CAD build for the part. Positions are in the model's coordinates, mm. Face numbers are marked on the shaded views. A direction names the side the tool comes from. Give positions to 0.01 mm unless a question says otherwise; leave off trailing zeros. Order: outer loops, then holes, each group sorted by start corner. A loop starts at its lowest first (then second) coordinate and runs counter-clockwise, first axis right, second up. Notation, with made-up numbers: (53, -26.5) -> (99, -26.5) arc R34 cw to (99, 6.5) -> close; hole circle Ø2 at (-37, -36). An arc over 180 degrees is marked (long way). Use one line per item in the form item = value. Start each with the question number.
1) Mould opens along Z. For the marked faces 4 and 5 say: pulls with the +Z half, pulls with the -Z half, needs draft (parallel to the pull), parting line crosses it, or undercut.
2) Cut at C-C, the plane x = 14.5. Give the cut face in (y, z).
3) Cut at D-D, the plane y = -45. Give the cut face in (x, z), and give its area (3 significant figures).
4) Probe line 1 (X direction, y = -50, z = 0); line 2 (Y direction, x = 14, z = 0); line 3 (X direction, y = 47.5, z = 1.5). List the from-to ranges inside material, lowest first.
5) Tool access for the marked faces 1, 2 and 3: list every direction of +Z, -Z, +X, -X, +Y, -Y with a clear straight run to the whole face (end or side of a thin tool).
6) Cut at B-B, the plane y = 16.5. Give the cut face in (x, z), and give its area (3 significant figures).
7) Drop flat-ended pins along their axis: P1, Ø8, axis at x = 81, y = -26, coming from the +Z side; P2, Ø6, axis at x = 52, y = 50.5, coming from the -Z side; P3, Ø6, axis at y = -35.5, z = -18.5, coming from the -X side. Give the stop position or say it passes through.
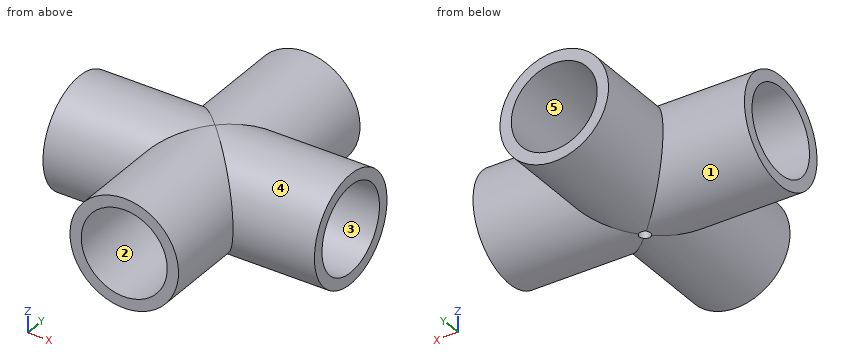
from build123d import *

# Parameters (mm, degrees)
SKETCH1_R                = 30.48
SKETCH1_R_2              = 24.13
BOSS_EXTRUDE1_DEPTH      = 152.4
BOSS_EXTRUDE2_DEPTH      = 76.2
BOSS_EXTRUDE2_DEPTH_BACK = 76.2
SKETCH2_R                = 30.48
SKETCH2_R_2              = 24.13
SKETCH4_R                = 3.175
CUT_EXTRUDE1_DEPTH       = 174.093126512


with BuildPart() as part:
    # Sketch1 → Boss-Extrude1 (new body)
    with BuildSketch(Plane(origin=(0, 0, 0), x_dir=(0, 0, -1), z_dir=(1, 0, 0))):
        with Locations(Location((0, 0, 0), (0, 0, 180))):
            Circle(SKETCH1_R)
        with Locations(Location((0, 0, 0), (0, 0, 180))):
            Circle(SKETCH1_R_2, mode=Mode.SUBTRACT)
    extrude(amount=BOSS_EXTRUDE1_DEPTH)

    # Sketch2 → Boss-Extrude2 (add, two sides: drawn at the far end of the back side and taken through both)
    with BuildSketch(Plane(origin=(0, 0, 0), x_dir=(1, 0, 0), z_dir=(0, 1, 0)).offset(-BOSS_EXTRUDE2_DEPTH_BACK)):
        with Locations(Location((76.2, 0, 0), (0, 0, 270))):
            Circle(SKETCH2_R)
        with Locations(Location((76.2, 0, 0), (0, 0, 270))):
            Circle(SKETCH2_R_2, mode=Mode.SUBTRACT)
    extrude(amount=BOSS_EXTRUDE2_DEPTH + BOSS_EXTRUDE2_DEPTH_BACK)

    # Sketch4 → Cut-Extrude1 (cut, through all)
    with BuildSketch(Plane.XY):
        with Locations(Location((76.2, 0, 0), (0, 0, 44.999999719))):
            Circle(SKETCH4_R)
    extrude(amount=-CUT_EXTRUDE1_DEPTH, mode=Mode.SUBTRACT)


solid = part.part
Result:
q1.face_4 = parting line crosses it
q1.face_5 = undercut
q2.outline = circle Ø60.96 at (0, 0); hole circle Ø48.26 at (0, 0)
q3.outline = circle Ø60.96 at (76.2, 0); hole circle Ø48.26 at (76.2, 0)
q3.area = 1,090 mm²
q4.line_1 = 45.72 to 52.07, 100.33 to 106.68
q4.line_2 = -30.48 to -24.13, 24.13 to 30.48
q4.line_3 = 45.76 to 52.12, 100.28 to 106.64
q5.face_1 = -X
q5.face_2 = -Y
q5.face_3 = +X
q6.outline = (0, -25.63) -> (59.7, -25.63) arc R30.48 ccw to (92.7, -25.63) -> (152.4, -25.63) -> (152.4, -17.61) -> (101.08, -17.61) arc R30.48 ccw to (101.08, 17.61) -> (152.4, 17.61) -> (152.4, 25.63) -> (92.7, 25.63) arc R30.48 ccw to (59.7, 25.63) -> (0, 25.63) -> (0, 17.61) -> (51.32, 17.61) arc R30.48 ccw to (51.32, -17.61) -> (0, -17.61) -> close; hole (59.7, -17.61) -> (92.7, -17.61) arc R24.13 ccw to (92.7, 17.61) -> (59.7, 17.61) arc R24.13 ccw to start
q6.area = 3,150 mm²
q7.P1 = 30.47
q7.P2 = -21.9
q7.P3 = 49.96
